from build123d import *

# Parameters (mm, degrees)
SKETCH1_R           = 11.25
BOSS_EXTRUDE1_DEPTH = 12
CHAMFER1_SIZE       = 0.5
BOSS_EXTRUDE2_DEPTH = 1
BOSS_EXTRUDE3_START = 0.5
SKETCH3_R           = 2
SKETCH3_R_2         = 1.5
BOSS_EXTRUDE3_DEPTH = 0.5


with BuildPart() as part:
    # Sketch1 → Boss-Extrude1 (new body)
    with BuildSketch(Plane(origin=(0, 0, 0), x_dir=(1, 0, 0), z_dir=(0, 1, 0))):
        with Locations(Location((0, 0, 0), (0, 0, 270))):
            Circle(SKETCH1_R)
    extrude(amount=BOSS_EXTRUDE1_DEPTH)

    # Chamfer1
    chamfer1_edges = [part.edges().sort_by_distance(p)[0] for p in [
        (0, 12, -11.25),
    ]]
    chamfer(chamfer1_edges, length=CHAMFER1_SIZE)

    # Sketch2 → Boss-Extrude2 (add)
    # profile 1 of 2: a face of its own
    with BuildSketch(Plane.XZ):
        with BuildLine():
            Line((-15.737008616, 2.388894786), (-10.514870422, 4))
            ThreePointArc((-10.514870422, 4), (-11.25, 0), (-10.514870422, -4))
            Line((-10.514870422, -4), (-15.737008616, -2.388894786))
            ThreePointArc((-15.737008616, -2.388894786), (-17.5, 0), (-15.737008616, 2.388894786))
        make_face()
        with BuildLine():
            Line((-15.963068014, 1.15), (-14.036931986, 1.15))
            ThreePointArc((-14.036931986, 1.15), (-13.5, 0), (-14.036931986, -1.15))
            Line((-14.036931986, -1.15), (-15.963068014, -1.15))
            ThreePointArc((-15.963068014, -1.15), (-16.5, 0), (-15.963068014, 1.15))
        make_face(mode=Mode.SUBTRACT)
    # profile 2 of 2: a face of its own
    with BuildSketch(Plane.XZ):
        with BuildLine():
            Line((15.737008616, -2.388894786), (10.514870422, -4))
            ThreePointArc((10.514870422, -4), (11.25, 0), (10.514870422, 4))
            Line((10.514870422, 4), (15.737008616, 2.388894786))
            ThreePointArc((15.737008616, 2.388894786), (17.5, 0), (15.737008616, -2.388894786))
        make_face()
        with BuildLine():
            Line((14.036931986, 1.15), (15.963068014, 1.15))
            ThreePointArc((15.963068014, 1.15), (16.5, 0), (15.963068014, -1.15))
            Line((15.963068014, -1.15), (14.036931986, -1.15))
            ThreePointArc((14.036931986, -1.15), (13.5, 0), (14.036931986, 1.15))
        make_face(mode=Mode.SUBTRACT)
    extrude(amount=-BOSS_EXTRUDE2_DEPTH)

    # Sketch3 → Boss-Extrude3 (add)
    # profile 1 of 2: a face of its own
    with BuildSketch(Plane.XZ.offset(BOSS_EXTRUDE3_START)):
        with Locations(Location((15, 0, 0), (0, 0, 270))):
            Circle(SKETCH3_R)
        with Locations(Location((15, 0, 0), (0, 0, 270))):
            Circle(SKETCH3_R_2, mode=Mode.SUBTRACT)
    # profile 2 of 2: a face of its own
    with BuildSketch(Plane.XZ.offset(BOSS_EXTRUDE3_START)):
        with Locations(Location((-15, 0, 0), (0, 0, 90))):
            Circle(SKETCH3_R)
        with Locations(Location((-15, 0, 0), (0, 0, 270))):
            Circle(SKETCH3_R_2, mode=Mode.SUBTRACT)
    extrude(amount=-BOSS_EXTRUDE3_DEPTH)


solid = part.part
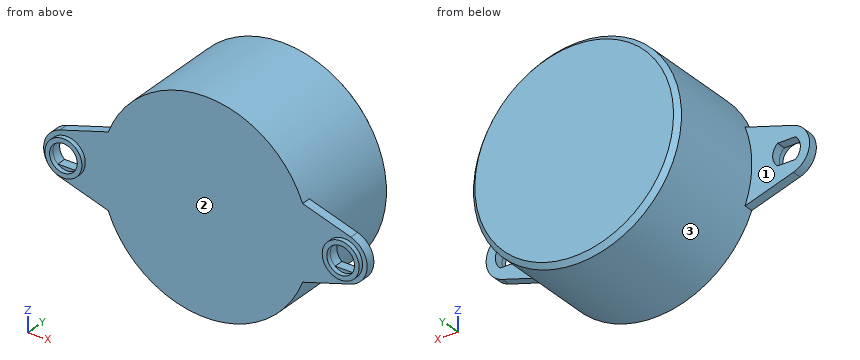
Read the model definition and answer for the solid it produces. Units are mm, in the model's axes. Face numbers are marked on the shaded views. Give positions to 0.01 mm unless a question says otherwise; leave off trailing zeros. Write each loop counter-clockwise with the first axis right and the second up, starting at its lowest first coordinate (ties: lowest second). Pieces come first, ordered by that corner, then holes. Notation, with made-up numbers: (46, 46.5) - (93, 46.5) arc R12 ccw to (93, 59.5) - close; hole circle Ø8 at (51.25, -28.5). An arc over 180 degrees is marked (long way). Use CSV: the item, a comma, the result in double quotes. Start each with the question number.
(1) Determine the mould class of the marked faces 1, 2 and 3 for opening direction X: +X half, -X half, draft (parallel to the pull), parting line (faces both ways), or undercut.
(2) Find section C-C (x = 15). Give the vertices of the cut face in (y, z).
(3) Find section B-B (x = 0). Give the vertices of the cut face in (y, z), plus the area to 3 significant figures.
(4) Consider line 1 along X through (y, z) = (-0.2, 0); line 2 along Z through (x, y) = (-15, -0.1); line 3 along Y through (x, z) = (-6.5, 3.25). Determine where each line is inside the solid, lowest interval first.
(5) Find section A-A (z = 0). Give the vertices of the cut face in (x, y).
(6) Find section D-D (y = 3). Give the vertices of the cut face in (x, z), plus the area to 3 significant figures.
(7) Given P1, Ø4, axis at x = 13, z = 1, coming from the +Y side; P2, Ø7.5, axis at x = -14.5, z = 2, coming from the +Y side; P3, Ø2.5, axis at x = 15, z = 0, coming from the +Y side; P4, Ø1.8, axis at x = -15, z = 0, coming from the +Y side, each flat-ended and moving along its own axis, determine where each tip first touches the part or whether it passes through.
Findings below:
1,face 1,"draft"
1,face 2,"undercut"
1,face 3,"parting line"
2,outline,"(-0.5, -2) - (0, -2) - (0, -2.62) - (1, -2.62) - (1, -1.15) - (0, -1.15) - (0, -1.5) - (-0.5, -1.5) - close; (-0.5, 1.5) - (0, 1.5) - (0, 1.15) - (1, 1.15) - (1, 2.62) - (0, 2.62) - (0, 2) - (-0.5, 2) - close"
3,outline,"(0, -11.25) - (11.5, -11.25) - (12, -10.75) - (12, 10.75) - (11.5, 11.25) - (0, 11.25) - close"
3,area,"270 mm2"
4,line 1,"-17 to -16.5, -13.5 to -13, 13 to 13.5, 16.5 to 17"
4,line 2,"-2 to -1.5, 1.5 to 2"
4,line 3,"0 to 12"
5,outline,"(-17.5, 0) - (-17, 0) - (-17, -0.5) - (-16.5, -0.5) - (-16.5, 1) - (-17.5, 1) - close; (-13.5, -0.5) - (-13, -0.5) - (-13, 0) - (13, 0) - (13, -0.5) - (13.5, -0.5) - (13.5, 1) - (11.25, 1) - (11.25, 11.5) - (10.75, 12) - (-10.75, 12) - (-11.25, 11.5) - (-11.25, 1) - (-13.5, 1) - close; (16.5, -0.5) - (17, -0.5) - (17, 0) - (17.5, 0) - (17.5, 1) - (16.5, 1) - close"
6,outline,"circle Ø22.5 at (0, 0)"
6,area,"398 mm2"
7,P1,"y = 11.71"
7,P2,"y = 11.86"
7,P3,"y = 1"
7,P4,"through"
